```python
from build123d import *

# Parameters (mm, degrees)
SKETCH3_R           = 1.6
BOSS_EXTRUDE1_DEPTH = 4


with BuildPart() as part:
    # Sketch3 → Boss-Extrude1 (new body)
    with BuildSketch(Plane(origin=(20.494506969, 51.628779219, -66.172927913), x_dir=(1, 0, 0), z_dir=(0, 0, 1))):
        with BuildLine():
            Line((-95, -35.45), (-76.606413565, -35.45))
            ThreePointArc((-76.606413565, -35.45), (-68.94960795, -36.890649791), (-61.222089264, -37.884429946))
            ThreePointArc((-61.222089264, -37.884429946), (-60.011397218, -38.080084438), (-58.833759818, -38.42246736))
            ThreePointArc((-58.833759818, -38.42246736), (-35.490101097, -45.151223745), (-11.481033396, -48.861645973))
            ThreePointArc((-11.481033396, -48.861645973), (-7.68167997, -53.388127631), (-12.188640475, -57.210617614))
            ThreePointArc((-12.188640475, -57.210617614), (-39.092131211, -53.124111692), (-65.141573254, -45.254936785))
            ThreePointArc((-65.141573254, -45.254936785), (-79.981953338, -42.810785721), (-95, -41.992843223))
            ThreePointArc((-95, -41.992843223), (-98.271421612, -38.721421612), (-95, -35.45))
        make_face()
        with Locations((-42.686731091, -46.672569756)):
            Circle(SKETCH3_R, mode=Mode.SUBTRACT)
        with Locations((-20.494506969, -51.628779219)):
            Circle(SKETCH3_R, mode=Mode.SUBTRACT)
    extrude(amount=BOSS_EXTRUDE1_DEPTH)


solid = part.part
```
CAD build for the part. Positions are in the model's coordinates, mm. Coordinates: 2 decimals unless noted, no trailing zeros. Write each loop counter-clockwise with the first axis right and the second up, starting at its lowest first coordinate (ties: lowest second). Pieces come first, ordered by that corner, then holes.
(1) Cut at D-D, the plane x = -17.5. List the corners of the cut face in (y, z), and give its area (3 significant figures).
(2) Two-plate mould, pull along X, no slides. Class faces 1 (the face through (-39.53, 13.55, -64.2)), 2 (the face through (-18.23, -1.58, -64.2)), 3 (the face through (-1.27, -0.97, -64.2)), 4 (the face through (-20.666, 5.437, -64.201)): +X half, -X half, draft (parallel to the pull), parting line (faces both ways), or undercut.
(3) Cut at A-A, the plane y = 0. List the corners of the cut face in (x, z).
(4) Drill centre lines: probe 1 along Y at (x, z) = (0, -65.1); probe 2 along Y at (x, z) = (-22, -65.9); probe 3 along Y at (x, z) = (-52.5, -65.45). Where is each one in solid material? Low to high.
(5) Flat gauge pin, fed straight in: pin 1 (2 mm diameter, centred on y = 1.5, z = -64.5, fed in from +X). Where does the tip first touch, or does it go through?
(6) Cut at C-C, the plane x = 0. List the corners of the cut face in (y, z), and give its area (3 significant figures).
(7) Cut at B-B, the plane z = -63.8. List the corners of the cut face in (x, y).
Geometry says:
1. outline: (-1.74, -66.17) - (7.05, -66.17) - (7.05, -62.17) - (-1.74, -62.17) - close
1. area: 35.1 mm2
2. face 1: +X half
2. face 2: -X half
2. face 3: undercut
2. face 4: undercut
3. outline: (-24.74, -66.17) - (-1.6, -66.17) - (-1.6, -62.17) - (-24.74, -62.17) - close; (1.6, -66.17) - (12.58, -66.17) - (12.58, -62.17) - (1.6, -62.17) - close
4. probe 1: y = -4.74 to -1.6, 1.6 to 3.79
4. probe 2: y = -0.69 to 3.37, 6.54 to 8.16
4. probe 3: y = 7.87 to 15.44
5. pin 1: stops at x = 12.37
6. outline: (-4.74, -66.17) - (-1.6, -66.17) - (-1.6, -62.17) - (-4.74, -62.17) - close; (1.6, -66.17) - (3.79, -66.17) - (3.79, -62.17) - (1.6, -62.17) - close
6. area: 21.3 mm2
7. outline: (-74.51, 9.64) arc R138.28 cw to (-44.65, 6.37) arc R190.95 ccw to (8.31, -5.58) arc R4.19 ccw to (9.01, 2.77) arc R190.95 cw to (-38.34, 13.21) arc R10 ccw to (-40.73, 13.74) arc R134.17 cw to (-56.11, 16.18) - (-74.51, 16.18) arc R3.27 ccw to start; hole circle Ø3.2 at (-22.19, 4.96); hole circle Ø3.2 at (0, 0)
